```python
from build123d import *

# Parameters (mm, degrees)
F0_W     = 30
F0_H     = 12
F1_DEPTH = 2
F2_W     = 30
F2_H     = 9
F3_DEPTH = 2.2
F4_W     = 30
F4_H     = 22
F4_H_2   = 9
F4_H_3   = 6
F5_DEPTH = 3
F6_R     = 2.5


with BuildPart() as f1:
    # F0 (on Top) → F1 (new body)
    with BuildSketch(Plane.XY):
        with Locations((15, -6)):
            Rectangle(F0_W, F0_H)
    extrude(amount=F1_DEPTH)

    # F2 (on face) → F3 (join)
    with BuildSketch(Plane.XY.offset(2)):
        with Locations((15, -6)):
            Rectangle(F2_W, F2_H)
    extrude(amount=F3_DEPTH)

    # F4 (on face) → F5 (join)
    with BuildSketch(Plane.XY.offset(4.2)):
        with Locations((15, -21.5)):
            Rectangle(F4_W, F4_H)
        with Locations((15, -6)):
            Rectangle(F4_W, F4_H_2)
        with Locations((15, 1.5)):
            Rectangle(F4_W, F4_H_3)
    extrude(amount=F5_DEPTH)

    # F6
    f6_edges = [f1.edges().sort_by_distance(p)[0] for p in [
        (0, -32.5, 5.7),
        (30, -32.5, 5.7),
        (30, 4.5, 5.7),
        (0, 4.5, 5.7),
    ]]
    fillet(f6_edges, radius=F6_R)


solid = f1.part
```
The listing builds one solid part. Answer for the finished solid, in the listing's coordinates (mm). A direction names the side the tool comes from. Round coordinates to 2 decimals unless told otherwise and drop trailing zeros. Loops run counter-clockwise (first coordinate to the right, second up) from the corner with the lowest first, then second, coordinate; pieces in that order, holes last.
1) A cutting plane is placed at A-A on x = 21.25. Determine the outline of the cut face in (y, z), plus the area to 3 significant figures.
Outcome:
outline: (-32.5, 4.2) - (-10.5, 4.2) - (-10.5, 2) - (-12, 2) - (-12, 0) - (0, 0) - (0, 2) - (-1.5, 2) - (-1.5, 4.2) - (4.5, 4.2) - (4.5, 7.2) - (-32.5, 7.2) - close
area: 155 mm2
2) A cutting plane is placed at D-D on x = 2. Determine the outline of the cut face in (y, z).
Outcome:
outline: (-32.45, 4.2) - (-10.5, 4.2) - (-10.5, 2) - (-12, 2) - (-12, 0) - (0, 0) - (0, 2) - (-1.5, 2) - (-1.5, 4.2) - (4.45, 4.2) - (4.45, 7.2) - (-32.45, 7.2) - close
3) A cutting plane is placed at C-C on y = -22. Determine the outline of the cut face in (x, z), plus the area to 3 significant figures.
Outcome:
outline: (0, 4.2) - (30, 4.2) - (30, 7.2) - (0, 7.2) - close
area: 90.0 mm2
4) Consider line 1 (Z direction, x = 7.5, y = -17.5); line 2 (Y direction, x = 16.5, z = 2.5); line 3 (Y direction, x = 24.75, z = 0.5). Determine where each line is inside the solid, lowest interval first.
Outcome:
line 1: z = 4.2 to 7.2
line 2: y = -10.5 to -1.5
line 3: y = -12 to 0
5) Given P1, Ø8, axis at x = 21, y = -22, coming from the -Z side; P2, Ø1.8, axis at x = 11, z = 3, coming from the +Y side; P3, Ø0.6, axis at x = 21.5, z = 0.5, coming from the -Y side, each flat-ended and moving along its own axis, determine where each tip first touches the part or whether it passes through.
Outcome:
P1: stops at z = 4.2
P2: stops at y = -1.5
P3: stops at y = -12
6) A cutting plane is placed at B-B on z = 1.5. Determine the outline of the cut face in (x, y), plus the area to 3 significant figures.
Outcome:
outline: (0, -12) - (30, -12) - (30, 0) - (0, 0) - close
area: 360 mm2
7) For faces 1 (the face through (15, -11, 2)), 2 (the face through (15, 2, 4.2)), 3 (the face through (15, 0, 1)), 4 (the face through (15, -12, 1)), 5 (the face through (0, -10, 4)), determine the directions among +Z, -Z, +X, -X, +Y, -Y from which every point of the face is accessible in a straight line to the end or side of a thin tool.
Outcome:
face 1: +X, -X, -Y
face 2: +X, -X, +Y
face 3: -Z, +X, -X, +Y
face 4: -Z, +X, -X, -Y
face 5: +Z, -Z, -X, +Y, -Y
8) For a pull along Z with two mould halves and no side action, classify faces 6 (the face through (1, -32, 6)), 7 (the face through (15, -10.5, 3)), 8 (the face through (15, -14, 7.2)) as released by +Z, released by -Z, zero draft, split by the parting line, or undercut.
Outcome:
face 6: zero draft
face 7: undercut
face 8: released by +Z
